Work out the finished part from the listing and answer in its coordinate system (mm). Face numbers are marked on the shaded views. A direction names the side the tool comes from. Coordinates: 2 decimals unless noted, no trailing zeros. Order: outer loops, then holes, each group sorted by start corner. A loop starts at its lowest first (then second) coordinate and runs counter-clockwise, first axis right, second up.
1. The part is cut by section A-A, the plane z = -40. Give the vertices of the cut face in (x, y).
2. Find the intervals of material crossed by probe 1 along Y at (x, z) = (7.75, -39); probe 2 along X at (y, z) = (9.75, -40); probe 3 along Z at (x, y) = (7.25, 10.75), in increasing order.
3. A tool of negligible diameter and unlimited length cuts with its end or side. For the marked faces 1, 2 and 3, from which of +Z, -Z, +X, -X, +Y, -Y can it reach the whole face along a straight path? Write none if from no direction.
4. The part is cut by section C-C, the plane y = 3. Give the vertices of the cut face in (x, z), then the cut area to 3 significant figures.
5. The part is cut by section D-D, the plane z = -12. Give the vertices of the cut face in (x, y), then the cut area to 3 significant figures.
6. The part is cut by section B-B, the plane x = 4.75. Give the vertices of the cut face in (y, z).
7. Flat-ended cylindrical pins translate along their axes: pin 1 Ø2.5 at (x, z) = (5.48, -40) entering from -Y; pin 2 Ø1.5 at (x, z) = (3.5, -16.5) entering from +Y; pin 3 Ø6 at (y, z) = (10.5, -36.5) entering from +X; pin 4 Ø1.6 at (x, y) = (5, 6.5) entering from +Z. Find the tip coordinate at first contact, or state that the pin passes through.
```python
from build123d import *

# Parameters (mm, degrees)
SKETCH1_W               = 10.962182916
SKETCH1_H               = 45
SKETCH1_R               = 1.25
BOSS_EXTRUDE1_DEPTH     = 5
SKETCH2_W               = 10.962182916
SKETCH2_H               = 2.5
BOSS_EXTRUDE2_DEPTH     = 8.2
SKETCH3_W               = 10.962182916
SKETCH3_H               = 5
BOSS_EXTRUDE3_DEPTH     = 5
CUT_EXTRUDE1_DEPTH      = 48.036256806
CUT_EXTRUDE1_DEPTH_BACK = 48.036256806
SKETCH4_R               = 1.6
SKETCH5_W               = 10.962182916
SKETCH5_H               = 13.2
BOSS_EXTRUDE4_DEPTH     = 5


with BuildPart() as part:
    # Sketch1 → Boss-Extrude1 (new body)
    with BuildSketch(Plane(origin=(0, 0, 0), x_dir=(1, 0, 0), z_dir=(0, 1, 0))):
        with Locations((5.481091458, 22.5)):
            Rectangle(SKETCH1_W, SKETCH1_H)
        with Locations(Location((5.481091458, 40, 0), (0, 0, 270))):
            Circle(SKETCH1_R, mode=Mode.SUBTRACT)
        with BuildLine():
            Line((7.081091458, 27.08548866), (7.081091458, 21.08548866))
            ThreePointArc((7.081091458, 21.08548866), (5.481091458, 19.48548866), (3.881091458, 21.08548866))
            Line((3.881091458, 21.08548866), (3.881091458, 27.08548866))
            ThreePointArc((3.881091458, 27.08548866), (5.481091458, 28.68548866), (7.081091458, 27.08548866))
        make_face(mode=Mode.SUBTRACT)
        with BuildLine():
            Line((3.881091458, 3.28548866), (3.881091458, 9.28548866))
            ThreePointArc((3.881091458, 9.28548866), (5.481091458, 10.88548866), (7.081091458, 9.28548866))
            Line((7.081091458, 9.28548866), (7.081091458, 3.28548866))
            ThreePointArc((7.081091458, 3.28548866), (5.481091458, 1.68548866), (3.881091458, 3.28548866))
        make_face(mode=Mode.SUBTRACT)
    extrude(amount=BOSS_EXTRUDE1_DEPTH)

    # Sketch2 → Boss-Extrude2 (add)
    with BuildSketch(Plane(origin=(0, 5, 0), x_dir=(1, 0, 0), z_dir=(0, 1, 0))):
        with Locations((5.481091458, 43.75)):
            Rectangle(SKETCH2_W, SKETCH2_H)
    extrude(amount=BOSS_EXTRUDE2_DEPTH)

    # Sketch3 → Boss-Extrude3 (add)
    with BuildSketch(Plane.XY.offset(-42.5)):
        with Locations((5.481091458, 10.7)):
            Rectangle(SKETCH3_W, SKETCH3_H)
    extrude(amount=BOSS_EXTRUDE3_DEPTH)

    # Sketch4 → Cut-Extrude1 (cut, two sides: drawn at the far end of the back side and taken through both)
    with BuildSketch(Plane.XZ.offset(-8.2).offset(-CUT_EXTRUDE1_DEPTH_BACK)):
        with Locations(Location((5.481091458, -40, 0), (0, 0, 270))):
            Circle(SKETCH4_R)
    extrude(amount=CUT_EXTRUDE1_DEPTH + CUT_EXTRUDE1_DEPTH_BACK, mode=Mode.SUBTRACT)

    # Sketch5 → Boss-Extrude4 (add)
    with BuildSketch(Plane(origin=(0, 0, -45), x_dir=(-1, 0, 0), z_dir=(0, 0, -1))):
        with Locations((-5.481091458, 6.6)):
            Rectangle(SKETCH5_W, SKETCH5_H)
    extrude(amount=BOSS_EXTRUDE4_DEPTH)


solid = part.part
```
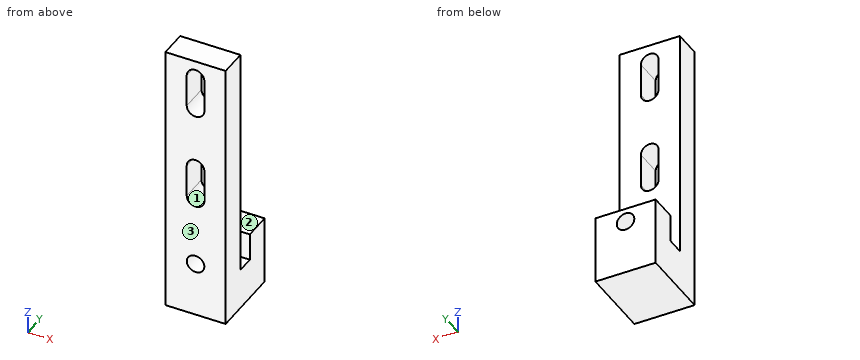
Geometry says:
1. outline: (0, 0) - (3.88, 0) - (3.88, 5) - (0, 5) - close; (0, 8.2) - (3.88, 8.2) - (3.88, 13.2) - (0, 13.2) - close; (7.08, 0) - (10.96, 0) - (10.96, 5) - (7.08, 5) - close; (7.08, 8.2) - (10.96, 8.2) - (10.96, 13.2) - (7.08, 13.2) - close
2. probe 1: y = 0 to 5, 8.2 to 13.2
2. probe 2: x = 0 to 3.88, 7.08 to 10.96
2. probe 3: z = -50 to -37.5
3. face 1: +Y, -Y
3. face 2: +Z, +X, -X, +Y
3. face 3: +Z, -Z, +X, -X, -Y
4. outline: (0, -50) - (10.96, -50) - (10.96, 0) - (0, 0) - close; hole circle Ø3.2 at (5.48, -40); hole (3.88, -27.09) arc R1.6 ccw to (7.08, -27.09) - (7.08, -21.09) arc R1.6 ccw to (3.88, -21.09) - close; hole (3.88, -9.29) arc R1.6 ccw to (7.08, -9.29) - (7.08, -3.29) arc R1.6 ccw to (3.88, -3.29) - close
4. area: 486 mm2
5. outline: (0, 0) - (10.96, 0) - (10.96, 5) - (0, 5) - close
5. area: 54.8 mm2
6. outline: (0, -50) - (13.2, -50) - (13.2, -41.42) - (8.2, -41.42) - (8.2, -42.5) - (5, -42.5) - (5, -41.42) - (0, -41.42) - close; (0, -38.58) - (5, -38.58) - (5, -28.51) - (0, -28.51) - close; (0, -19.66) - (5, -19.66) - (5, -10.71) - (0, -10.71) - close; (0, -1.86) - (5, -1.86) - (5, 0) - (0, 0) - close; (8.2, -38.58) - (13.2, -38.58) - (13.2, -37.5) - (8.2, -37.5) - close
7. pin 1: passes through
7. pin 2: stops at y = 5
7. pin 3: stops at x = 10.96
7. pin 4: stops at z = -42.5
